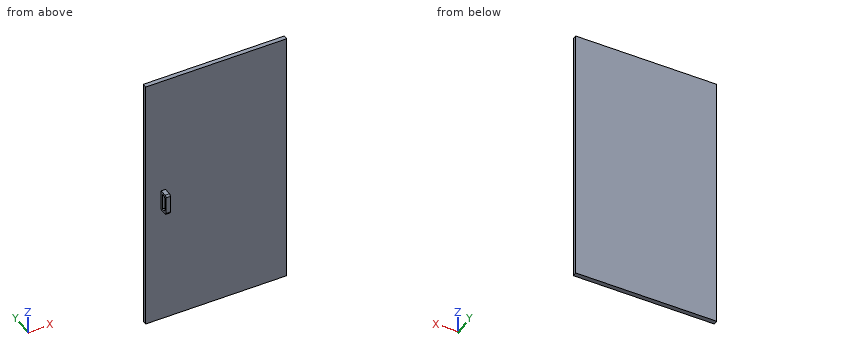
from build123d import *

# Parameters (mm, degrees)
F0_W     = 406.4
F0_H     = 762
F1_DEPTH = 12.7
F3_DEPTH = 25.4
F5_DEPTH = 86.36
F6_R     = 5.08


with BuildPart() as f1:
    # F0 (on Front) → F1 (new body)
    with BuildSketch(Plane.XZ):
        Rectangle(F0_W, F0_H)
    extrude(amount=F1_DEPTH)

    # F2 (on face) → F3 (join)
    with BuildSketch(Plane.XZ.offset(12.7)):
        Polygon((-146.05, -30.14731), (-146.05, 30.14731), (-158.75, 30.14731), (-158.75, 0), (-158.75, -30.14731), align=None)
    extrude(amount=F3_DEPTH)

    # F4 (on face) → F5 (cut)
    with BuildSketch(Plane.YZ.offset(-146.05)):
        Polygon((-31.75, 23.79731), (-31.75, 0), (-31.75, -23.79731), (-19.05, -23.79731), (-19.05, 23.79731), align=None)
    extrude(amount=-F5_DEPTH, mode=Mode.SUBTRACT)

    # F6
    f6_edges = [f1.edges().sort_by_distance(p)[0] for p in [
        (-152.4, -38.1, 30.14731),
        (-152.4, -38.1, -30.14731),
        (-152.4, -31.75, 23.79731),
        (-152.4, -31.75, -23.79731),
    ]]
    fillet(f6_edges, radius=F6_R)


solid = f1.part
CAD build for the part. Positions are in the model's coordinates, mm. Round coordinates to 2 decimals unless told otherwise and drop trailing zeros. Order: outer loops, then holes, each group sorted by start corner. A loop starts at its lowest first (then second) coordinate and runs counter-clockwise, first axis right, second up. Notation, with made-up numbers: M -10.75,10 L 26.25,10 A19 cw 26.25,42 Z; hole C 18,31.5 d9. An arc over 180 degrees is marked long. Use one line per item in the form item = value.
Q1. Saw through at B-B on z = 40.5. Give the cut face in (x, y).
Recorded:
outline = M -203.2,-12.7 L 203.2,-12.7 L 203.2,0 L -203.2,0 Z
Q2. Probe L1, parallel to Y at x = -61, z = -69. List the from-to ranges inside material, lowest first.
Recorded:
L1 = -12.7 to 0
Q3. Flat gauge pins, fed straight in: P1, Ø6.5, axis at x = -150.5, y = -19, coming from the -Z side; P2, Ø4, axis at x = -154.5, y = -23.5, coming from the +Z side; P3, Ø6, axis at x = 83, z = -83.5, coming from the -Y side. Where does each tip first touch, or does it go through?
Recorded:
P1 = -30.15
P2 = 30.15
P3 = -12.7
Q4. Saw through at A-A on x = 176.5. Give the cut face in (y, z), then the cut area to 3 significant figures.
Recorded:
outline = M -12.7,-381 L 0,-381 L 0,381 L -12.7,381 Z
area = 9,680 mm^2
